Autodesk Inventor part; units mm, degrees
ref_plane "YZ Plane" through (0, 0, 0) normal (1, 0, 0) x (0, 1, 0)
ref_plane "XZ Plane" through (0, 0, 0) normal (0, 1, 0) x (-1, 0, 0)
ref_plane "XY Plane" through (0, 0, 0) normal (0, 0, 1) x (1, 0, 0)
sketch "Sketch1" plane through (0, 0, 0) normal (1, 0, 0) x (0, 1, 0)
  line L0 (0, 0) -> (120, 0)
  line L1 (120, 0) -> (120, -99)
  line L2 (120, -99) -> (0, -99)
  line L3 (0, -99) -> (0, 0)
  dimension "d0" = 120
  dimension "d1" = 99
extrude "Extrusion1" add sketch "Sketch1" along normal blind 6
sketch "Sketch2" plane through (6, 0, 0) normal (1, 0, 0) x (0, 0, -1)
  line L0 (0, 120) -> (0, 0)
  line L1 (0, 0) -> (99, 0)
  line L2 (99, 0) -> (99, 120)
  line L3 (99, 120) -> (0, 120)
  line L4 (0, 120) -> (0, 0)
  line L5 (0, 15) -> (5.75, 15)
  line L6 (5.75, 15) -> (5.75, 45)
  line L7 (5.75, 45) -> (0, 45)
  line L8 (0, 45) -> (0, 15)
  line L9 (0, 75) -> (5.75, 75)
  line L10 (5.75, 75) -> (5.75, 105)
  line L11 (5.75, 105) -> (0, 105)
  line L12 (0, 105) -> (0, 75)
  line L13 (99, 15) -> (93.25, 15)
  line L14 (93.25, 15) -> (93.25, 45)
  line L15 (93.25, 45) -> (99, 45)
  line L16 (99, 45) -> (99, 15)
  line L17 (99, 75) -> (93.25, 75)
  line L18 (93.25, 75) -> (93.25, 105)
  line L19 (93.25, 105) -> (99, 105)
  line L20 (99, 105) -> (99, 75)
  line L21 (-12.0657, 60) -> (104.2665, 60)
  line L22 (99, 120) -> (0, 120)
  dimension "d5" = 5.75
  dimension "d6" = 5.75
  dimension "d8" = 30
  dimension "d9" = 30
  dimension "d22" = 60
  dimension "d23" = 15
  dimension "d24" = 15
extrude "Extrusion2" cut sketch "Sketch2" against normal up to next contours L11 L10 L9 L0 | L2 L17 L18 L19 | L7 L6 L5 L0 | L2 L13 L14 L15
sketch "Sketch3" plane through (6, 0, 0) normal (1, 0, 0) x (0, 0, -1)
  circle A0 centre (79, 10) radius 2.3
  circle A1 centre (79, 110) radius 2.3
  line L0 (99, 105) -> (99, 120)
  line L1 (99, 120) -> (0, 120)
  line L2 (99, 0) -> (99, 15)
  line L3 (0, 0) -> (99, 0)
  dimension "d13" = 20
  dimension "d14" = 10
  dimension "d15" = 4.6
  dimension "d17" = 10
  dimension "d18" = 20
  dimension "d19" = 4.6
extrude "Extrusion3" cut sketch "Sketch3" against normal up to next
properties part number "Side"
For this review, take the finished solid that the model builds, in its own axes (mm). A direction names the side the tool comes from. Give positions to 0.01 mm unless a question says otherwise; leave off trailing zeros. Write each loop counter-clockwise with the first axis right and the second up, starting at its lowest first coordinate (ties: lowest second). Pieces come first, ordered by that corner, then holes.
Item 1: Machinability: for faces 1 (the face through (3, 75, -96)), 2 (the face through (3.042, 10.691, -81.194)), 3 (the face through (3, 90, -5.75)), which of the approach directions +Z, -Z, +X, -X, +Y, -Y give a long, thin tool a straight path to every point of the face, cutting with its end or side? Answer none if there is none.
Item 2: Insertion check: P1, Ø1.8, axis at x = 1.5, y = 27, coming from the -Z side; P2, Ø2, axis at x = 1.5, y = 37, coming from the +Z side. Each pin has a flat end and moves straight along its axis. Give the tip position at first contact, or say it passes through.
Item 3: Take a section at D-D (y = 34). Give the boundary of the cut face in (x, z), and give its area (3 significant figures).
Item 4: Take a section at B-B (x = 4.8). Give the boundary of the cut face in (y, z).
Item 5: Wall thickness on probe 1 along Y at (x, z) = (2.15, -79); probe 2 along Z at (x, y) = (4.6, 96); probe 3 along Z at (x, y) = (2.9, 112): over which ranges is each line inside the solid? List them lowest first.
Item 6: Take a section at A-A (y = 10). Give the boundary of the cut face in (x, z), and give its area (3 significant figures).
Item 7: Take a section at C-C (z = -79). Give the boundary of the cut face in (x, y).
Item 8: The part is to be moulded in two halves that separate along Y. For faces 4 (the face through (3, 112, 0)), 5 (the face through (3, 30, -93.25)), say which applies: +Y half, -Y half, draft (parallel to the pull), parting line (faces both ways), or undercut.
Established:
1. face 1: -Z, +X, -X
1. face 2: +X, -X
1. face 3: +Z, +X, -X
2. P1: stops at z = -93.25
2. P2: stops at z = -5.75
3. outline: (0, -93.25) - (6, -93.25) - (6, -5.75) - (0, -5.75) - close
3. area: 525 mm2
4. outline: (0, -99) - (15, -99) - (15, -93.25) - (45, -93.25) - (45, -99) - (75, -99) - (75, -93.25) - (105, -93.25) - (105, -99) - (120, -99) - (120, 0) - (105, 0) - (105, -5.75) - (75, -5.75) - (75, 0) - (45, 0) - (45, -5.75) - (15, -5.75) - (15, 0) - (0, 0) - close; hole circle Ø4.6 at (10, -79); hole circle Ø4.6 at (110, -79)
5. probe 1: y = 0 to 7.7, 12.3 to 107.7, 112.3 to 120
5. probe 2: z = -93.25 to -5.75
5. probe 3: z = -99 to -80.14, -77.86 to 0
6. outline: (0, -99) - (6, -99) - (6, -81.3) - (0, -81.3) - close; (0, -76.7) - (6, -76.7) - (6, 0) - (0, 0) - close
6. area: 566 mm2
7. outline: (0, 0) - (6, 0) - (6, 7.7) - (0, 7.7) - close; (0, 12.3) - (6, 12.3) - (6, 107.7) - (0, 107.7) - close; (0, 112.3) - (6, 112.3) - (6, 120) - (0, 120) - close
8. face 4: draft
8. face 5: undercut
